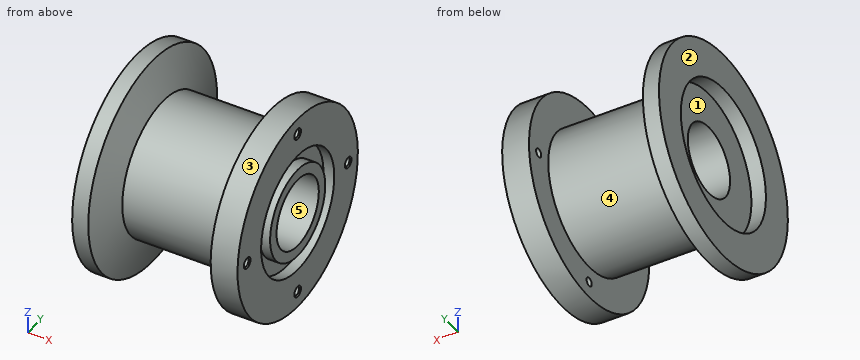
from build123d import *

# Parameters (mm, degrees)
HOLE_WIZARD_M21_D           = 1.6
HOLE_WIZARD_M21_DEPTH       = 5
HOLE_WIZARD_M21_CSINK_D     = 2.05
HOLE_WIZARD_M21_CSINK_ANGLE = 90
PATTERN_CIRCULAR_1_COUNT    = 4


with BuildPart() as part:
    # Эскиз1 → Повернуть1 (revolve)
    with BuildSketch(Plane.XY, mode=Mode.PRIVATE) as revolve_1_sk:
        Polygon((0, 20), (0, 13.2), (2.7, 13.2), (2.7, 6.56), (30, 6.56), (30, 8.56), (28, 8.56), (28, 11.36), (30, 11.36), (30, 18.675), (25, 18.675), (25, 12.7), (4.956029105, 12.7), (3, 20), align=None)
    revolve(revolve_1_sk.sketch.rotate(Axis((-29.041238464, 0, 0), (1, 0, 0)), 90), axis=Axis((-29.041238464, 0, 0), (1, 0, 0)))

    # Отверстие обработанное метчиком M21
    with Locations(Plane(origin=(30, 0, 0), x_dir=(0, 0, -1), z_dir=(1, 0, 0))):
        with Locations((0, 15.675)):
            hole_wizard_m21 = CounterSinkHole(HOLE_WIZARD_M21_D / 2, HOLE_WIZARD_M21_CSINK_D / 2, depth=HOLE_WIZARD_M21_DEPTH, counter_sink_angle=HOLE_WIZARD_M21_CSINK_ANGLE)

    # Круговой массив1: Отверстие обработанное метчиком M21 ×4 about axis
    pattern_circular_1_axis = Axis((0, 0, 0), (1, 0, 0))
    for i in range(1, PATTERN_CIRCULAR_1_COUNT):
        add(hole_wizard_m21.rotate(pattern_circular_1_axis, i * 360 / PATTERN_CIRCULAR_1_COUNT), mode=Mode.SUBTRACT)


solid = part.part
Check sheet for the modelled part. Datum: model origin and axes. Units: mm. Face numbers are marked on the shaded views. A direction names the side the tool comes from. Round coordinates to 2 decimals unless told otherwise and drop trailing zeros. Loops run counter-clockwise (first coordinate to the right, second up) from the corner with the lowest first, then second, coordinate; pieces in that order, holes last. Notation, with made-up numbers: M 9.25,41 L 57.25,41 A23 cw 57.25,72 Z; hole C 39.25,-14 d5. An arc over 180 degrees is marked long. One line per question, with ' | ' between items. Start each with the question number.
Item 1: Section check A-A (x = 17). Record the boundary of the cut face in (y, z), and give its area (3 significant figures).
Item 2: Section check D-D (x = 26.5). Record the boundary of the cut face in (y, z) (3 decimals), and give its area (3 significant figures).
Item 3: Gauge pin test, flat ends, axial feed: pin 1 Ø5 at (x, z) = (14.5, 12) entering from -Y; pin 2 Ø13 at (y, z) = (-4, 4) entering from -X; pin 3 Ø1 at (y, z) = (15.675, 0) entering from +X. Record the tip position at first contact, or that the pin passes through.
Item 4: Set-up check for the marked faces 4 and 5: record each of +Z, -Z, +X, -X, +Y, -Y from which the full face is reachable in a straight line by a thin tool's end or side.
Item 5: Release check for a two-part mould opening along Y. For the marked faces 1, 2 and 3 record: released by +Y, released by -Y, zero draft, split by the parting line, or undercut.
Item 6: Section check B-B (y = 0). State how many separate pieces and enclosed holes the cut face has, and give its area (3 significant figures).
Item 7: Scan lines: probe 1 along Y at (x, z) = (27.3, 0) (3 decimals); probe 2 along Y at (x, z) = (29.05, 0) (3 decimals); probe 3 along Z at (x, y) = (29.5, 3.5). Record each from-to range of solid material in increasing order.
Worked out:
1) outline: C 0,0 d25.4; hole C 0,0 d13.12 | area: 372 mm^2
2) outline: C 0,0 d37.35; hole C -15.675,0 d1.6; hole C 0,0 d13.12; hole C 0,-15.675 d1.6; hole C 0,15.675 d1.6; hole C 15.675,0 d1.6 | area: 952 mm^2
3) pin 1: y = -8.43 | pin 2: x = 2.7 | pin 3: x = 4.29
4) face 4: none | face 5: +X, -X
5) face 1: undercut | face 2: zero draft | face 3: split by the parting line
6) separate pieces: 4 | enclosed holes: 0 | area: 423 mm^2
7) probe 1: -18.675 to -16.475, -14.875 to -6.56, 6.56 to 14.875, 16.475 to 18.675 | probe 2: -18.675 to -16.475, -14.875 to -11.36, -8.56 to -6.56, 6.56 to 8.56, 11.36 to 14.875, 16.475 to 18.675 | probe 3: -18.34 to -10.81, -7.81 to -5.55, 5.55 to 7.81, 10.81 to 18.34
